Model file for the job. Use its own axes, mm. A direction names the side the tool comes from. Round coordinates to 2 decimals unless told otherwise and drop trailing zeros. Order: outer loops, then holes, each group sorted by start corner. A loop starts at its lowest first (then second) coordinate and runs counter-clockwise, first axis right, second up. Notation, with made-up numbers: M 42.5,25 L 60.5,25 A22 cw 60.5,49 Z; hole C 71.5,32 d9. An arc over 180 degrees is marked long. Return JSON: item names as keys, results as strings. Group by question number.
Item 1: Which spindle directions (+Z, -Z, +X, -X, +Y, -Y) get a long thin tool onto all of the face, cutting with end or side? Do faces 1 (the face through (2.48, 8.21, -0.33)), 2 (the face through (2.562, -3.451, 1.452)), 3 (the face through (2.54, -3.45, -1.49)), 4 (the face through (-2.54, -3.45, 1.49)), 5 (the face through (0, -3, 2.944)). Say none if no direction does.
Item 2: Slice it at A-A on y = 1. Write the cut outline in (x, z).
Item 3: Probe line 1 along X through (y, z) = (17.25, -2); line 2 along Z through (x, y) = (1.25, -5.25); line 3 along Z through (x, y) = (-2.25, -4). List the from-to ranges inside material, lowest first.
Item 4: Pull direction X, two halves, no side cores. Call faces 6 (the face through (2, 2.1, -2)), 7 (the face through (-2.562, -3.451, -1.452)), 8 (the face through (-1.2, 10.1, 1.8)), 9 (the face through (1.2, 10.1, 1.8)): pulls with the +X half, pulls with the -X half, needs draft (parallel to the pull), parting line crosses it, or undercut.
Item 5: Pin check, flat tips, straight feed: pin 1 Ø1 at (y, z) = (14, -0.5) entering from +X; pin 2 Ø1 at (x, y) = (-0.5, 14.5) entering from +Z; pin 3 Ø2 at (x, y) = (1.5, 1) entering from -Z. Stop position of each tip, or through.
Item 6: Slice it at B-B on y = 7. Write the cut outline in (x, z).
from build123d import *

# Parameters (mm, degrees)
SKETCH1_R           = 3.15
BOSS_EXTRUDE1_DEPTH = 2.1
SKETCH2_R           = 2.5
BOSS_EXTRUDE3_DEPTH = 16
SKETCH8_OUTSIDE_W   = 12.334
SKETCH8_OUTSIDE_H   = 12.334
CUT_EXTRUDE5_DEPTH  = 8
BOSS_EXTRUDE4_DEPTH = 7


with BuildPart() as part:
    # Sketch1 → Boss-Extrude1 (new body)
    with BuildSketch(Plane(origin=(0, 0, 0), x_dir=(1, 0, 0), z_dir=(0, 1, 0))):
        with Locations(Location((0, 0, 0), (0, 0, 270))):
            Circle(SKETCH1_R)
    extrude(amount=BOSS_EXTRUDE1_DEPTH)

    # Sketch2 → Boss-Extrude3 (add)
    with BuildSketch(Plane(origin=(0, 2.1, 0), x_dir=(1, 0, 0), z_dir=(0, 1, 0))):
        with Locations(Location((0, 0, 0), (0, 0, 270))):
            Circle(SKETCH2_R)
    extrude(amount=BOSS_EXTRUDE3_DEPTH)

    # Sketch8 outside → Cut-Extrude5 (cut)
    with BuildSketch(Plane(origin=(0, 18.1, 0), x_dir=(1, 0, 0), z_dir=(0, 1, 0))):
        Rectangle(SKETCH8_OUTSIDE_W, SKETCH8_OUTSIDE_H)
        with BuildLine():
            ThreePointArc((-0.874874584, -1.914509945), (-0.872847435, -1.898524314), (-0.871608771, -1.882458342))
            ThreePointArc((-0.871608771, -1.882458342), (-1.021648634, -1.589716304), (-1.350264969, -1.574844682))
            ThreePointArc((-1.350264969, -1.574844682), (-1.364364531, -1.582645457), (-1.378063464, -1.591130087))
            ThreePointArc((-1.378063464, -1.591130087), (-1.575187068, -1.691186219), (-1.789333192, -1.746053167))
            ThreePointArc((-1.789333192, -1.746053167), (-1.889436652, -1.637206179), (-1.982929527, -1.522631086))
            ThreePointArc((-1.982929527, -1.522631086), (-1.898144875, -1.318473041), (-1.771053556, -1.137595344))
            ThreePointArc((-1.771053556, -1.137595344), (-1.760705725, -1.125243335), (-1.750977775, -1.112397452))
            ThreePointArc((-1.750977775, -1.112397452), (-1.718931045, -0.785009505), (-1.987340492, -0.594835296))
            ThreePointArc((-1.987340492, -0.594835296), (-2.003419215, -0.593774926), (-2.019530629, -0.593506449))
            ThreePointArc((-2.019530629, -0.593506449), (-2.239455986, -0.571105958), (-2.449270481, -0.501486836))
            ThreePointArc((-2.449270481, -0.501486836), (-2.474635746, -0.355798906), (-2.491342985, -0.20886614))
            ThreePointArc((-2.491342985, -0.20886614), (-2.309641425, -0.082955507), (-2.104935538, 0.00049774))
            ThreePointArc((-2.104935538, 0.00049774), (-2.089552388, 0.005294452), (-2.074423707, 0.010841769))
            ThreePointArc((-2.074423707, 0.010841769), (-1.870464994, 0.268932266), (-1.99344945, 0.574030094))
            ThreePointArc((-1.99344945, 0.574030094), (-2.006402454, 0.583614948), (-2.019811088, 0.592551293))
            ThreePointArc((-2.019811088, 0.592551293), (-2.192713451, 0.73029641), (-2.331581698, 0.902298023))
            ThreePointArc((-2.331581698, 0.902298023), (-2.274155475, 1.038572006), (-2.208772648, 1.17121233))
            ThreePointArc((-2.208772648, 1.17121233), (-1.987843141, 1.178899814), (-1.770515359, 1.138432796))
            ThreePointArc((-1.770515359, 1.138432796), (-1.754980932, 1.134151287), (-1.739254769, 1.130638805))
            ThreePointArc((-1.739254769, 1.130638805), (-1.428139525, 1.237489942), (-1.366652294, 1.560644985))
            ThreePointArc((-1.366652294, 1.560644985), (-1.37236709, 1.5757112), (-1.378815798, 1.590478186))
            ThreePointArc((-1.378815798, 1.590478186), (-1.449799889, 1.799834828), (-1.4736322, 2.019609634))
            ThreePointArc((-1.4736322, 2.019609634), (-1.351646909, 2.103203644), (-1.224932602, 2.179439161))
            ThreePointArc((-1.224932602, 2.179439161), (-1.034918706, 2.066462775), (-0.873969064, 1.914923482))
            ThreePointArc((-0.873969064, 1.914923482), (-0.86321543, 1.902923103), (-0.851884731, 1.891466009))
            ThreePointArc((-0.851884731, 1.891466009), (-0.532389846, 1.813153306), (-0.30595269, 2.05176612))
            ThreePointArc((-0.30595269, 2.05176612), (-0.302614872, 2.067530279), (-0.300056235, 2.083439494))
            ThreePointArc((-0.300056235, 2.083439494), (-0.246585106, 2.297938405), (-0.14781489, 2.495709457))
            ThreePointArc((-0.14781489, 2.495709457), (-0.073939789, 2.498989364), (0, 2.500082986))
            ThreePointArc((0, 2.500082986), (0.073939789, 2.498989364), (0.14781489, 2.495709457))
            ThreePointArc((0.14781489, 2.495709457), (0.246585106, 2.297938405), (0.300056235, 2.083439494))
            ThreePointArc((0.300056235, 2.083439494), (0.302614872, 2.067530279), (0.30595269, 2.05176612))
            ThreePointArc((0.30595269, 2.05176612), (0.532389846, 1.813153306), (0.851884731, 1.891466009))
            ThreePointArc((0.851884731, 1.891466009), (0.86321543, 1.902923103), (0.873969064, 1.914923482))
            ThreePointArc((0.873969064, 1.914923482), (1.034918706, 2.066462775), (1.224932602, 2.179439161))
            ThreePointArc((1.224932602, 2.179439161), (1.351646909, 2.103203644), (1.4736322, 2.019609634))
            ThreePointArc((1.4736322, 2.019609634), (1.449799889, 1.799834828), (1.378815798, 1.590478186))
            ThreePointArc((1.378815798, 1.590478186), (1.37236709, 1.5757112), (1.366652294, 1.560644985))
            ThreePointArc((1.366652294, 1.560644985), (1.428139525, 1.237489942), (1.739254769, 1.130638805))
            ThreePointArc((1.739254769, 1.130638805), (1.754980932, 1.134151287), (1.770515359, 1.138432796))
            ThreePointArc((1.770515359, 1.138432796), (1.987843141, 1.178899814), (2.208772648, 1.17121233))
            ThreePointArc((2.208772648, 1.17121233), (2.274155475, 1.038572006), (2.331581698, 0.902298023))
            ThreePointArc((2.331581698, 0.902298023), (2.192713451, 0.73029641), (2.019811088, 0.592551293))
            ThreePointArc((2.019811088, 0.592551293), (2.006402454, 0.583614948), (1.99344945, 0.574030094))
            ThreePointArc((1.99344945, 0.574030094), (1.870464994, 0.268932266), (2.074423707, 0.010841769))
            ThreePointArc((2.074423707, 0.010841769), (2.089552388, 0.005294452), (2.104935538, 0.00049774))
            ThreePointArc((2.104935538, 0.00049774), (2.309641425, -0.082955507), (2.491342985, -0.20886614))
            ThreePointArc((2.491342985, -0.20886614), (2.474635746, -0.355798906), (2.449270481, -0.501486836))
            ThreePointArc((2.449270481, -0.501486836), (2.239455986, -0.571105958), (2.019530629, -0.593506449))
            ThreePointArc((2.019530629, -0.593506449), (2.003419215, -0.593774926), (1.987340492, -0.594835296))
            ThreePointArc((1.987340492, -0.594835296), (1.718931045, -0.785009505), (1.750977775, -1.112397452))
            ThreePointArc((1.750977775, -1.112397452), (1.760705725, -1.125243335), (1.771053556, -1.137595344))
            ThreePointArc((1.771053556, -1.137595344), (1.898144875, -1.318473041), (1.982929527, -1.522631086))
            ThreePointArc((1.982929527, -1.522631086), (1.889436652, -1.637206179), (1.789333192, -1.746053167))
            ThreePointArc((1.789333192, -1.746053167), (1.575187069, -1.691186219), (1.378063467, -1.591130087))
            ThreePointArc((1.378063467, -1.591130087), (1.364364533, -1.582645456), (1.350264971, -1.574844682))
            ThreePointArc((1.350264971, -1.574844682), (1.021648634, -1.589716304), (0.871608771, -1.882458343))
            ThreePointArc((0.871608771, -1.882458343), (0.872847435, -1.898524314), (0.874874584, -1.914509946))
            ThreePointArc((0.874874584, -1.914509946), (0.884000739, -2.135384701), (0.844949955, -2.352971421))
            ThreePointArc((0.844949955, -2.352971421), (0.704354772, -2.398812058), (0.561295258, -2.436259955))
            ThreePointArc((0.561295258, -2.436259955), (0.410807386, -2.274326806), (0.299070887, -2.083581165))
            ThreePointArc((0.299070887, -2.083581165), (0.292133749, -2.069037237), (0.284489859, -2.05485201))
            ThreePointArc((0.284489859, -2.05485201), (0, -1.88969941), (-0.284489859, -2.054852009))
            ThreePointArc((-0.284489859, -2.054852009), (-0.292133749, -2.069037237), (-0.299070887, -2.083581165))
            ThreePointArc((-0.299070887, -2.083581165), (-0.410807386, -2.274326806), (-0.561295258, -2.436259955))
            ThreePointArc((-0.561295258, -2.436259955), (-0.704354772, -2.398812058), (-0.844949955, -2.352971421))
            ThreePointArc((-0.844949955, -2.352971421), (-0.884000739, -2.135384701), (-0.874874584, -1.914509945))
        make_face(mode=Mode.SUBTRACT)
    extrude(amount=-CUT_EXTRUDE5_DEPTH, mode=Mode.SUBTRACT)

    # Sketch9 → Boss-Extrude4 (add)
    with BuildSketch(Plane.XZ):
        Polygon((3.4, 0), (1.7, 2.944486373), (-1.7, 2.944486373), (-3.4, 0), (-1.7, -2.944486373), (1.7, -2.944486373), align=None)
    extrude(amount=BOSS_EXTRUDE4_DEPTH)


solid = part.part
Output values:
{
 "1": {"face 1": "+Y", "face 2": "+Z, +X, -Y", "face 3": "-Z, +X, -Y", "face 4": "+Z, -X, -Y", "face 5": "+Z, +X, -X, -Y"},
 "2": {"outline": "C 0,0 d6.3"},
 "3": {"line 1": "-1.47 to -0.96, -0.32 to 0.32, 0.96 to 1.47", "line 2": "-2.94 to 2.94", "line 3": "-1.99 to 1.99"},
 "4": {"face 6": "needs draft", "face 7": "pulls with the -X half", "face 8": "undercut", "face 9": "undercut"},
 "5": {"pin 1": "x = 2.33", "pin 2": "z = 2.44", "pin 3": "z = -3.11"},
 "6": {"outline": "C 0,0 d5"}
}
